```python
from build123d import *


with BuildPart() as part:
    # 掃出1: sweep along a path in 草圖1
    with BuildLine(Plane.XY) as sweep_1_path:
        Line((1.088041762, -2.111111111), (3.664982778, -7.111111111))
        ThreePointArc((3.664982778, -7.111111111), (0, -13.123105626), (-3.664982778, -7.111111111))
        Line((-3.664982778, -7.111111111), (-0.555555556, -1.077936111))
        ThreePointArc((-0.555555556, -1.077936111), (-0.140873421, 0.034166823), (0, 1.212678125))
        Line((0, 1.212678125), (0, 31.212678125))
        Line((0, 31.212678125), (-1.5, 33.810754337))
        ThreePointArc((-1.5, 33.810754337), (-4.5, 33.810754337), (-3, 31.212678125))
    # 草圖3 → 掃出1 (sweep)
    with BuildSketch(Plane(origin=(-3, 31.212678125, 0), x_dir=(0, 0, -1), z_dir=(1, 0, 0))):
        with BuildLine():
            Line((-0.901387819, 1.5), (0.901387819, 1.5))
            ThreePointArc((0.901387819, 1.5), (1.237436867, 1.237436867), (1.5, 0.901387819))
            Line((1.5, 0.901387819), (1.5, -0.901387819))
            ThreePointArc((1.5, -0.901387819), (1.237436867, -1.237436867), (0.901387819, -1.5))
            Line((0.901387819, -1.5), (-0.901387819, -1.5))
            ThreePointArc((-0.901387819, -1.5), (-1.237436867, -1.237436867), (-1.5, -0.901387819))
            Line((-1.5, -0.901387819), (-1.5, 0.901387819))
            ThreePointArc((-1.5, 0.901387819), (-1.237436867, 1.237436867), (-0.901387819, 1.5))
        make_face()
    sweep(path=sweep_1_path.line, transition=Transition.RIGHT)


solid = part.part
```
The model under review builds one solid part; all positions refer to its coordinate system, in mm. A direction names the side the tool comes from. Give positions to 0.01 mm unless a question says otherwise; leave off trailing zeros. Write each loop counter-clockwise with the first axis right and the second up, starting at its lowest first coordinate (ties: lowest second). Pieces come first, ordered by that corner, then holes. Notation, with made-up numbers: (57, 72) - (67, 72) arc R13 cw to (67, 91) - close; hole circle Ø9 at (25.25, 2.25). An arc over 180 degrees is marked (long way). Answer in a Markdown table with one row per item. Add a question column.
1. Wall thickness on line 1 along X through (y, z) = (25.5, 0.2); line 2 along X through (y, z) = (-7, -1.25); line 3 along Y through (x, z) = (-4, -0.8): over which ranges is each line inside the solid? List them lowest first. Write a range as [from, to].
2. Draft analysis for pull direction X (two halves, no side actions). For faces 1 (the cylindrical face through (-3.192, -3.483, 1.233)), 2 (the cylindrical face through (0.414, 32.979, -1.233)), 3 (the flat face through (-3, 31, 0)), state which applies: +X half, -X half, draft (parallel to the pull), parting line (faces both ways), or undercut.
3. Tool access review of faces 4 (the cylindrical face through (-1.6, 0.38, 0.01)), 5 (the flat face through (1.5, 17, 0)), 6 (the cylindrical face through (-1.9, 32.01, 1.23)): name each direction out of +Z, -Z, +X, -X, +Y, -Y from which nothing blocks a thin tool from reaching the whole face with its end or side.
4. Insertion check: P1, Ø1.4, axis at y = 10.5, z = 0, coming from the +X side; P2, Ø0.5, axis at y = 23, z = 0, coming from the -X side. Each pin has a flat end and moves straight along its axis. Give the tip position at first contact, or say it passes through.
5. We need section A-A on y = 2. Write out the cut boundary in (x, z).
Ans:
| question | item | result |
|---|---|---|
| 1 | line 1 | x = [-1.5, 1.5] |
| 1 | line 2 | x = [-4.96, -2.23], [2.23, 4.96] |
| 1 | line 3 | y = [-12.95, -4.49], [29.87, 36.02] |
| 2 | face 1 | -X half |
| 2 | face 2 | +X half |
| 2 | face 3 | undercut |
| 3 | face 4 | +Z, -Z, -X |
| 3 | face 5 | +Z, -Z, +X, +Y |
| 3 | face 6 | +Z |
| 4 | P1 | stops at x = 1.5 |
| 4 | P2 | stops at x = -1.5 |
| 5 | outline | (-1.5, -0.9) arc R1.75 ccw to (-0.9, -1.5) - (0.9, -1.5) arc R1.75 ccw to (1.5, -0.9) - (1.5, 0.9) arc R1.75 ccw to (0.9, 1.5) - (-0.9, 1.5) arc R1.75 ccw to (-1.5, 0.9) - close |
